The drawing under review shows one solid part. Ordinate dimensions are in mm from its lowest x, y, z. Round coordinates to 2 decimals unless told otherwise and drop trailing zeros. Order: outer loops, then holes, each group sorted by start corner. A loop starts at its lowest first (then second) coordinate and runs counter-clockwise, first axis right, second up. Notation, with made-up numbers: (-9, -39) -> (19, -39) arc R25 cw to (19, -12) -> close; hole circle Ø11 at (5.25, 71). An arc over 180 degrees is marked (long way). Put each result on its own line as item: value. Start each with the question number.
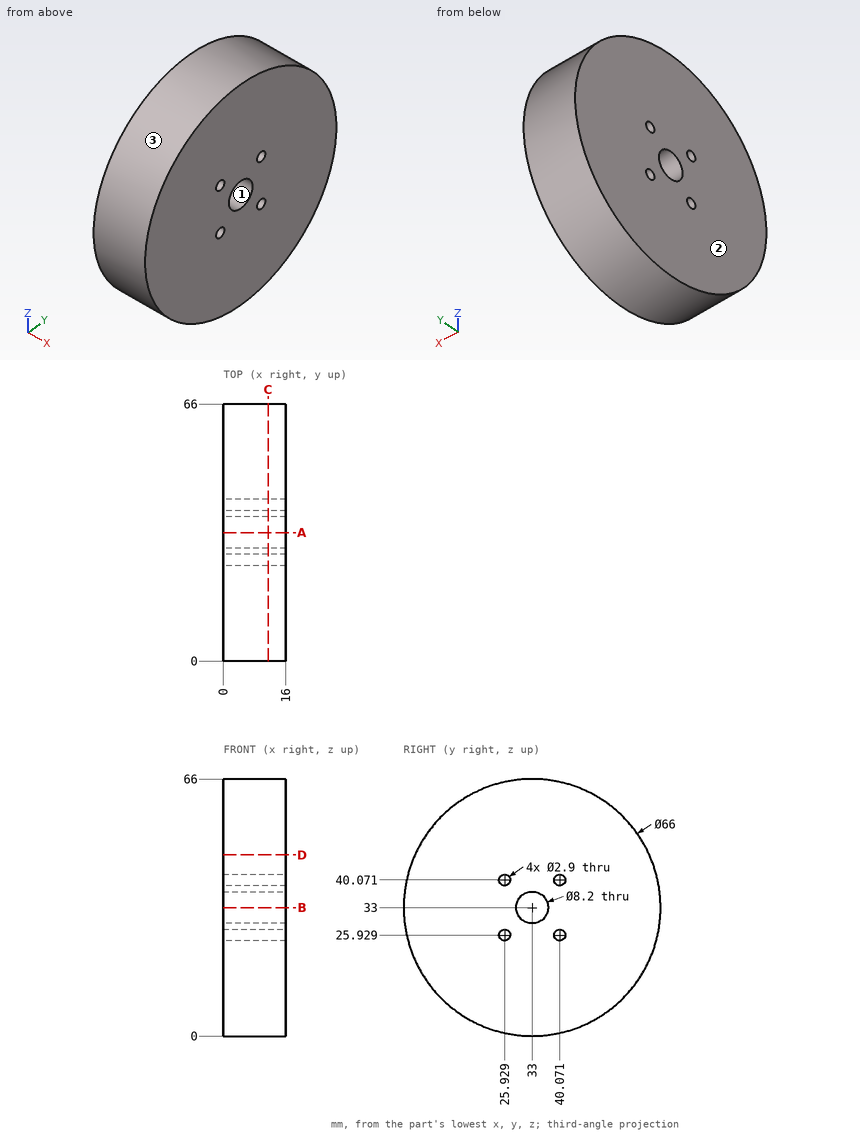
Item 1: Consider section A-A, the plane y = 33. Write out the cut boundary in (x, z), plus the area to 3 significant figures.
Item 2: Consider section D-D, the plane z = 46.5. Write out the cut boundary in (x, y), plus the area to 3 significant figures.
Item 3: For L1, parallel to Z at x = 9, y = 31.5; L2, parallel to Y at x = 7, z = 12; L3, parallel to Y at x = 15.25, z = 13, list the stretches that pass through material, from the lowest coordinate up.
Item 4: Mouldability with a two-part tool opening along Y and no side actions: class the marked faces 1, 2 and 3 as +Y half, -Y half, draft (parallel to the pull), parting line (faces both ways), or undercut.
Item 5: Insertion check: pin 1 Ø4 at (x, z) = (7, 46) entering from +Y; pin 2 Ø5 at (x, y) = (3.5, 36.5) entering from +Z; pin 3 Ø2 at (x, z) = (6, 56) entering from +Y; pin 4 Ø5 at (y, z) = (33, 33) entering from -X. Each pin has a flat end and moves straight along its axis. Give the tip position at first contact, or say it passes through.
Item 6: Consider section C-C, the plane x = 11.5. Write out the cut boundary in (y, z), plus the area to 3 significant figures.
Evaluation:
1. outline: (0, 0) -> (16, 0) -> (16, 28.9) -> (0, 28.9) -> close; (0, 37.1) -> (16, 37.1) -> (16, 66) -> (0, 66) -> close
1. area: 925 mm^2
2. outline: (0, 2.89) -> (16, 2.89) -> (16, 63.11) -> (0, 63.11) -> close
2. area: 964 mm^2
3. L1: z = 0.03 to 29.18, 36.82 to 65.97
3. L2: y = 7.54 to 58.46
3. L3: y = 6.75 to 59.25
4. face 1: undercut
4. face 2: draft
4. face 3: parting line
5. pin 1: stops at y = 64.11
5. pin 2: stops at z = 65.98
5. pin 3: stops at y = 57.6
5. pin 4: passes through
6. outline: circle Ø66 at (33, 33); hole circle Ø2.9 at (25.93, 25.93); hole circle Ø2.9 at (25.93, 40.07); hole circle Ø8.2 at (33, 33); hole circle Ø2.9 at (40.07, 25.93); hole circle Ø2.9 at (40.07, 40.07)
6. area: 3,340 mm^2
